```python
from build123d import *

# Parameters (mm, degrees)
BOSS_EXTRUDE1_START = 0.3
BOSS_EXTRUDE1_DEPTH = 4.7
SKETCH2_W           = 1.75
SKETCH2_H           = 0.5
BOSS_EXTRUDE2_DEPTH = 0.3
FILLET1_R           = 0.5


with BuildPart() as part:
    # Sketch1 → Boss-Extrude1 (new body)
    with BuildSketch(Plane(origin=(0, 0, 0), x_dir=(1, 0, 0), z_dir=(0, 1, 0)).offset(BOSS_EXTRUDE1_START)):
        with BuildLine():
            Line((-3.15, 2.7), (3.15, 2.7))
            ThreePointArc((3.15, 2.7), (3.503553391, 2.553553391), (3.65, 2.2))
            Line((3.65, 2.2), (3.65, -2.2))
            ThreePointArc((3.65, -2.2), (3.503553391, -2.553553391), (3.15, -2.7))
            Line((3.15, -2.7), (-3.15, -2.7))
            ThreePointArc((-3.15, -2.7), (-3.503553391, -2.553553391), (-3.65, -2.2))
            Line((-3.65, -2.2), (-3.65, 2.2))
            ThreePointArc((-3.65, 2.2), (-3.503553391, 2.553553391), (-3.15, 2.7))
        make_face()
    extrude(amount=BOSS_EXTRUDE1_DEPTH)

    # Sketch2 → Boss-Extrude2 (add)
    with BuildSketch(Plane(origin=(0, 0, 0), x_dir=(1, 0, 0), z_dir=(0, 1, 0))):
        with Locations((3.625, -1.27)):
            Rectangle(SKETCH2_W, SKETCH2_H)
        with Locations((3.625, 1.27)):
            Rectangle(SKETCH2_W, SKETCH2_H)
        with Locations((-3.625, 1.27)):
            Rectangle(SKETCH2_W, SKETCH2_H)
        with Locations((-3.625, -1.27)):
            Rectangle(SKETCH2_W, SKETCH2_H)
    extrude(amount=BOSS_EXTRUDE2_DEPTH)

    # Fillet1
    fillet1_edges = [part.edges().sort_by_distance(p)[0] for p in [
        (3.503553391, 5, -2.553553391),
        (0, 5, -2.7),
        (-3.503553391, 5, -2.553553391),
        (-3.65, 5, 0),
        (-3.503553391, 5, 2.553553391),
        (0, 5, 2.7),
        (3.503553391, 5, 2.553553391),
        (3.65, 5, 0),
    ]]
    fillet(fillet1_edges, radius=FILLET1_R)


solid = part.part
```
Build history of the part. All positions in model axes, mm. Round coordinates to 2 decimals unless told otherwise and drop trailing zeros. Order: outer loops, then holes, each group sorted by start corner. A loop starts at its lowest first (then second) coordinate and runs counter-clockwise, first axis right, second up. Notation, with made-up numbers: (-19.5, 78) - (26.5, 78) arc R13 ccw to (26.5, 103) - close; hole circle Ø5 at (-39.75, 40). An arc over 180 degrees is marked (long way). Use a Markdown table: item, result.
1) Wall check: L1, parallel to Y at x = -3, z = -0.3; L2, parallel to X at y = 1.95, z = 0.6. Give the ranges that are in metal, low to high.
Recorded:
| item | result |
|---|---|
| L1 | y = 0.3 to 5 |
| L2 | x = -3.65 to 3.65 |
2) Saw through at C-C on x = 1.5. Write the cut outline in (y, z), and give its area (3 significant figures).
Recorded:
| item | result |
|---|---|
| outline | (0.3, -2.7) - (4.5, -2.7) arc R0.5 ccw to (5, -2.2) - (5, 2.2) arc R0.5 ccw to (4.5, 2.7) - (0.3, 2.7) - close |
| area | 25.3 mm² |
3) Saw through at A-A on y = 3.35. Write the cut outline in (x, z), and give its area (3 significant figures).
Recorded:
| item | result |
|---|---|
| outline | (-3.65, -2.2) arc R0.5 ccw to (-3.15, -2.7) - (3.15, -2.7) arc R0.5 ccw to (3.65, -2.2) - (3.65, 2.2) arc R0.5 ccw to (3.15, 2.7) - (-3.15, 2.7) arc R0.5 ccw to (-3.65, 2.2) - close |
| area | 39.2 mm² |
4) Saw through at B-B on z = -0.8. Write the cut outline in (x, y).
Recorded:
| item | result |
|---|---|
| outline | (-3.65, 0.3) - (3.65, 0.3) - (3.65, 4.5) arc R0.5 ccw to (3.15, 5) - (-3.15, 5) arc R0.5 ccw to (-3.65, 4.5) - close |
5) Pull direction X, two halves, no side cores. Call faces 1 (the face through (-3.65, 2, 0)), 2 (the face through (3.65, 2, 0)), 3 (the face through (0, 5, 0)), 4 (the face through (0, 0.3, 0)): pulls with the +X half, pulls with the -X half, needs draft (parallel to the pull), parting line crosses it, or undercut.
Recorded:
| item | result |
|---|---|
| face 1 | pulls with the -X half |
| face 2 | pulls with the +X half |
| face 3 | needs draft |
| face 4 | undercut |
6) Flat gauge pins, fed straight in: pin 1 Ø1.3 at (y, z) = (3, -1) entering from +X; pin 2 Ø3 at (y, z) = (3.5, -0.5) entering from -X. Where does each tip first touch, or does it go through?
Recorded:
| item | result |
|---|---|
| pin 1 | stops at x = 3.65 |
| pin 2 | stops at x = -3.65 |
7) Saw through at D-D on z = 1.4. Write the cut outline in (x, y), and give its area (3 significant figures).
Recorded:
| item | result |
|---|---|
| outline | (-4.5, 0) - (-2.75, 0) - (-2.75, 0.3) - (2.75, 0.3) - (2.75, 0) - (4.5, 0) - (4.5, 0.3) - (3.65, 0.3) - (3.65, 4.5) arc R0.5 ccw to (3.15, 5) - (-3.15, 5) arc R0.5 ccw to (-3.65, 4.5) - (-3.65, 0.3) - (-4.5, 0.3) - close |
| area | 35.3 mm² |
